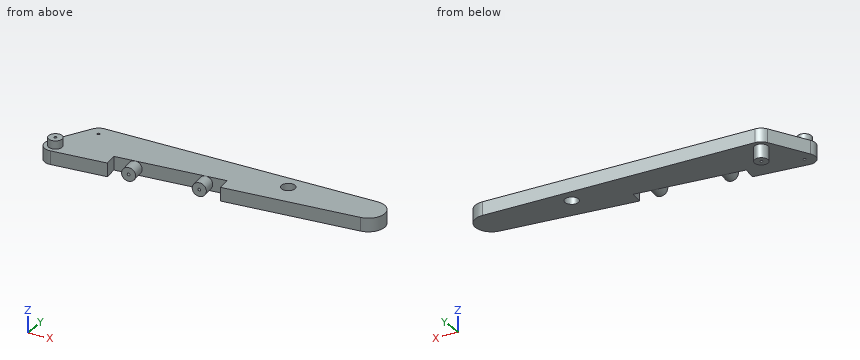
```python
from build123d import *

# Parameters (mm, degrees)
SKETCH3_R           = 2.5
BOSS_EXTRUDE1_DEPTH = 5
BOSS_EXTRUDE2_START = -10
SKETCH4_R           = 2.5
SKETCH4_R_2         = 0.5
BOSS_EXTRUDE2_DEPTH = 10
SKETCH5_R           = 2.5
SKETCH5_R_2         = 0.5
BOSS_EXTRUDE3_DEPTH = 8
SKETCH6_R           = 2.5
CUT_EXTRUDE1_DEPTH  = 5
CUT_EXTRUDE2_DEPTH  = 5
SKETCH8_R           = 2.5
SKETCH8_R_2         = 0.5
BOSS_EXTRUDE4_DEPTH = 5


with BuildPart() as part:
    # Sketch3 → Boss-Extrude1 (new body)
    with BuildSketch(Plane.XY):
        with BuildLine():
            Line((-11.551452097, -11.771319146), (-3.449219334, 2.025558191))
            ThreePointArc((-3.449219334, 2.025558191), (-2.00867995, 3.459075723), (-0.049634206, 3.999692044))
            Line((-0.049634206, 3.999692044), (100.92554869, 5.252744283))
            ThreePointArc((100.92554869, 5.252744283), (106.990382731, -0.40721355), (101.604045304, -6.716310453))
            Line((101.604045304, -6.716310453), (-7.699535894, -17.776555117))
            ThreePointArc((-7.699535894, -17.776555117), (-11.469136318, -15.956497778), (-11.551452097, -11.771319146))
        make_face()
        with Locations((-8.102232763, -13.796877337)):
            Circle(SKETCH3_R, mode=Mode.SUBTRACT)
        Circle(SKETCH3_R, mode=Mode.SUBTRACT)
    extrude(amount=BOSS_EXTRUDE1_DEPTH)

    # Sketch4 → Boss-Extrude2 (add)
    with BuildSketch(Plane.XY.offset(5).offset(BOSS_EXTRUDE2_START)):
        Circle(SKETCH4_R)
        Circle(SKETCH4_R_2, mode=Mode.SUBTRACT)
    extrude(amount=BOSS_EXTRUDE2_DEPTH)

    # Sketch5 → Boss-Extrude3 (add)
    with BuildSketch(Plane(origin=(0, 0, 0), x_dir=(-1, 0, 0), z_dir=(0, 0, -1))):
        with Locations((8.102232763, -13.796877337)):
            Circle(SKETCH5_R)
        with Locations((8.102232763, -13.796877337)):
            Circle(SKETCH5_R_2, mode=Mode.SUBTRACT)
    extrude(amount=-BOSS_EXTRUDE3_DEPTH)

    # Sketch6 → Cut-Extrude1 (cut)
    with BuildSketch(Plane(origin=(0, 0, 0), x_dir=(-1, 0, 0), z_dir=(0, 0, -1))):
        with Locations((-71, -0.524973847)):
            Circle(SKETCH6_R)
    extrude(amount=-CUT_EXTRUDE1_DEPTH, mode=Mode.SUBTRACT)

    # Sketch7 → Cut-Extrude2 (cut)
    with BuildSketch(Plane(origin=(0, 0, 0), x_dir=(-1, 0, 0), z_dir=(0, 0, -1))):
        Polygon((-52.217542839, -11.713647177), (-12.42076504, -15.740615868), (-11.91482349, -10.740615868), (-51.711601289, -6.713647177), align=None)
    extrude(amount=-CUT_EXTRUDE2_DEPTH, mode=Mode.SUBTRACT)

    # Sketch8 → Boss-Extrude4 (add)
    # profile 1 of 2: a face of its own
    with BuildSketch(Plane(origin=(1.196569763, -11.825177849, 0), x_dir=(0.9949194449683489, 0.10067421727469462, 0), z_dir=(0.10067421727469462, -0.9949194449683489, 0))):
        with Locations(Location((18.272986478, 2.5, 0), (0, 0, 270))):
            Circle(SKETCH8_R)
        with Locations((18.272986478, 2.5)):
            Circle(SKETCH8_R_2, mode=Mode.SUBTRACT)
    # profile 2 of 2: a face of its own
    with BuildSketch(Plane(origin=(1.196569763, -11.825177849, 0), x_dir=(0.9949194449683489, 0.10067421727469462, 0), z_dir=(0.10067421727469462, -0.9949194449683489, 0))):
        with Locations(Location((43.272986478, 2.5, 0), (0, 0, 270))):
            Circle(SKETCH8_R)
        with Locations((43.272986478, 2.5)):
            Circle(SKETCH8_R_2, mode=Mode.SUBTRACT)
    extrude(amount=BOSS_EXTRUDE4_DEPTH)


solid = part.part
```
Work out the finished part from the listing and answer in its coordinate system (mm). Round coordinates to 2 decimals unless told otherwise and drop trailing zeros. Write each loop counter-clockwise with the first axis right and the second up, starting at its lowest first coordinate (ties: lowest second). Pieces come first, ordered by that corner, then holes. Notation, with made-up numbers: (87.25, -16.75) - (119.25, -16.75) arc R22 cw to (119.25, 5.25) - close; hole circle Ø1 at (8, 80.25). An arc over 180 degrees is marked (long way). Return JSON: item names as keys, results as strings. Group by question number.
Q1. Each of these flat-tipped pins is pushed along its axis until it touches: pin 1 Ø7 at (x, y) = (35, -10) entering from -Z; pin 2 Ø10 at (x, y) = (39.5, -15) entering from -Z; pin 3 Ø12 at (x, y) = (6.5, -8.5) entering from +Z. Where does it stop, or does it pass through?
Q2. The part is cut by section C-C on x = 58.5. Write down the section's boundary in (y, z), then the cut area to 3 significant figures.
Q3. The part is cut by section D-D on x = 28. Write down the section's boundary in (y, z), then the cut area to 3 significant figures.
Q4. The part is cut by section A-A on x = 71. Write down the section's boundary in (y, z), then the cut area to 3 significant figures.
Q5. The part is cut by section B-B on z = -3.75. Write down the section's boundary in (x, y).
Q6. Find the intervals of material crossed by L1, parallel to X at y = -14, z = 0.5; L2, parallel to Z at x = 80, y = -8; L3, parallel to X at y = -1.25, z = 3.5, in increasing order.
Solved:
{
 "1": {"pin 1": "z = 0", "pin 2": "z = 0.17", "pin 3": "z = 5"},
 "2": {"outline": "(-11.08, 0) - (4.73, 0) - (4.73, 5) - (-11.08, 5) - close", "area": "79.0 mm²"},
 "3": {"outline": "(-9.11, 0) - (4.35, 0) - (4.35, 5) - (-9.11, 5) - close", "area": "67.3 mm²"},
 "4": {"outline": "(-9.81, 0) - (-3.02, 0) - (-3.02, 5) - (-9.81, 5) - close; (1.98, 0) - (4.88, 0) - (4.88, 5) - (1.98, 5) - close", "area": "48.5 mm²"},
 "5": {"outline": "circle Ø5 at (0, 0); hole circle Ø1 at (0, 0)"},
 "6": {"L1": "-12.1 to -8.56, -7.65 to 12.24, 18.28 to 21.29", "L2": "0 to 5", "L3": "-5.37 to 68.61, 73.39 to 106.98"}
}
